Autodesk Inventor part; units mm, degrees
ref_plane "YZ Plane" through (0, 0, 0) normal (1, 0, 0) x (0, 1, 0)
ref_plane "XZ Plane" through (0, 0, 0) normal (0, 1, 0) x (-1, 0, 0)
ref_plane "XY Plane" through (0, 0, 0) normal (0, 0, 1) x (1, 0, 0)
sketch "Boceto1" plane through (0, 0, 0) normal (0, 1, 0) x (-1, 0, 0)
  circle A0 centre (0, 0) radius 4.5
  dimension "d0" = 9
extrude "Extrusión1" add sketch "Boceto1" along normal blind 1.6
sketch "Boceto2" plane through (0, 1.6, 0) normal (0, 1, 0) x (1, 0, 0)
  circle A0 centre (0, 0) radius 2.5
  dimension "d3" = 5
extrude "Extrusión2" add sketch "Boceto2" along normal blind 8
fillet "Empalme1" radius 0.4 1 edges at (4.5, 0, 0)
fillet "Empalme2" radius 0.2 1 edges at (4.5, 1.6, 0)
sketch "Boceto3" plane through (0, 0, 0) normal (0, -1, 0) x (1, 0, 0)
  line L0 (-1.7321, 0) -> (-0.866, 1.5)
  line L1 (-0.866, 1.5) -> (0.866, 1.5)
  line L2 (0.866, 1.5) -> (1.7321, 0)
  line L3 (1.7321, 0) -> (0.866, -1.5)
  line L4 (0.866, -1.5) -> (-0.866, -1.5)
  line L5 (-0.866, -1.5) -> (-1.7321, 0)
  point P0 (0, 0)
  point P1 (0, 0)
  dimension "d8" = 3
extrude "Extrusión3" cut sketch "Boceto3" against normal blind 2.5
chamfer "Chaflán1" distance 0.5 angle 45 1 edges at (-2.5, 9.6, 0)
thread "Rosca2"
properties part number "Perno M5x8cabeza plana_" material "Hierro, gris"
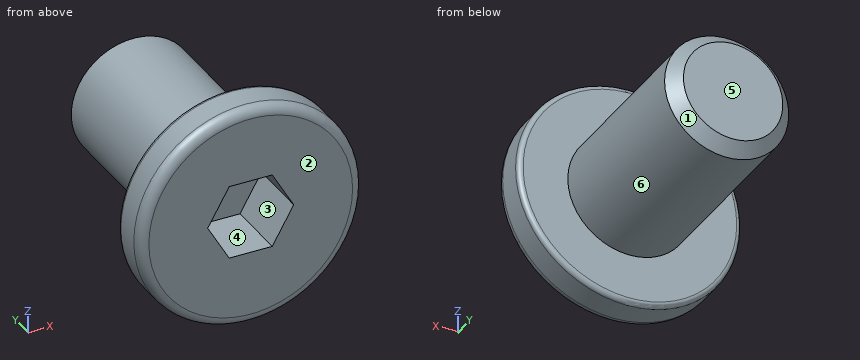
For this review, take the finished solid that the model builds, in its own axes (mm). Face numbers are marked on the shaded views. A direction names the side the tool comes from. Give positions to 0.01 mm unless a question says otherwise; leave off trailing zeros. Write each loop counter-clockwise with the first axis right and the second up, starting at its lowest first coordinate (ties: lowest second). Pieces come first, ordered by that corner, then holes. Notation, with made-up numbers: M 60.5,45 L 112.5,45 A18 cw 112.5,76 Z; hole C 18.5,35.5 d10. An arc over 180 degrees is marked long. One line per item, written item: value.
1) For line 1 (Z direction, x = 0, y = 2.25); line 2 (Z direction, x = -1.5, y = 5); line 3 (Z direction, x = 0, y = 6.75), list the stretches that pass through material, from the lowest coordinate up. Write a range as from..to.
Results are:
line 1: z = -2.5..-1.5, 1.5..2.5
line 2: z = -2..2
line 3: z = -2.5..2.5
2) The part is to be moulded in two halves that separate along Z. For the marked faces 1, 2 and 3, say which applies: +Z half, -Z half, draft (parallel to the pull), parting line (faces both ways), or undercut.
Results are:
face 1: parting line
face 2: draft
face 3: undercut
3) For P1, Ø1, axis at y = 5, z = 0.5, coming from the -X side; P2, Ø4, axis at x = 3.5, y = 7, coming from the +Z side; P3, Ø1, axis at x = 1, y = 3.5, coming from the +Z side, all flat-tipped, find the tip position at first contact; note any pin that passes through.
Results are:
P1: stops at x = -2.5
P2: stops at z = 2
P3: stops at z = 2.45
4) For the marked faces 4, 5 and 6, list the 3-axis set-ups (+Z, -Z, +X, -X, +Y, -Y) from which the entire face can be reached by the end or side of a thin tool; tool diameter is ignored.
Results are:
face 4: -Y
face 5: +Z, -Z, +X, -X, +Y
face 6: +Y
5) Take a section at A-A, the plane x = 0. Write out the cut boundary in (y, z).
Results are:
outline: M 0,-4.1 A0.4 ccw 0.4,-4.5 L 1.4,-4.5 A0.2 ccw 1.6,-4.3 L 1.6,-2.5 L 9.1,-2.5 L 9.6,-2 L 9.6,2 L 9.1,2.5 L 1.6,2.5 L 1.6,4.3 A0.2 ccw 1.4,4.5 L 0.4,4.5 A0.4 ccw 0,4.1 L 0,1.5 L 2.5,1.5 L 2.5,-1.5 L 0,-1.5 Z
6) Take a section at B-B, the plane y = 8. Write out the cut boundary in (x, z), then the cut area to 3 significant figures.
Results are:
outline: C 0,0 d5
area: 19.6 mm²
